from build123d import *

# Parameters (mm, degrees)
BOSS_EXTRUDE1_DEPTH = 12


with BuildPart() as part:
    # Sketch1 → Boss-Extrude1 (new body)
    with BuildSketch(Plane.XY):
        with BuildLine():
            Line((0.477214368, -2.672855337), (26.843355259, 7.215507779))
            ThreePointArc((26.843355259, 7.215507779), (36.953291517, 0.789364626), (27.989636176, -7.157899677))
            Line((27.989636176, -7.157899677), (15.076637928, -4.54511037))
            ThreePointArc((15.076637928, -4.54511037), (14.494851923, -4.485141012), (13.912410709, -4.538371753))
            Line((13.912410709, -4.538371753), (-14.128816251, -12.448152272))
            ThreePointArc((-14.128816251, -12.448152272), (-15.750958715, -12.635893161), (-17.350003272, -12.304759779))
            Line((-17.350003272, -12.304759779), (-32.894889614, -7.121812332))
            ThreePointArc((-32.894889614, -7.121812332), (-37.600806958, 2.472956777), (-27.935809428, 7.032899219))
            Line((-27.935809428, 7.032899219), (-1.504706088, -2.679457675))
            ThreePointArc((-1.504706088, -2.679457675), (-0.513152862, -2.854165557), (0.477214368, -2.672855337))
        make_face()
        with BuildLine():
            Line((-28.280719883, 6.094263625), (-1.849616543, -3.618093269))
            ThreePointArc((-1.849616543, -3.618093269), (-0.509821597, -3.854160008), (0.82837082, -3.609172135))
            Line((0.82837082, -3.609172135), (27.194511712, 6.279190981))
            ThreePointArc((27.194511712, 6.279190981), (35.956456468, 0.709866915), (28.187955173, -6.177762148))
            Line((28.187955173, -6.177762148), (15.274956925, -3.564972841))
            ThreePointArc((15.274956925, -3.564972841), (14.477361985, -3.485090396), (13.679767045, -3.564972841))
            Line((13.679767045, -3.564972841), (-14.400299195, -11.485709022))
            ThreePointArc((-14.400299195, -11.485709022), (-15.71642918, -11.636427946), (-17.012660358, -11.363116652))
            Line((-17.012660358, -11.363116652), (-32.578589422, -6.173153179))
            ThreePointArc((-32.578589422, -6.173153179), (-36.657051163, 2.142313468), (-28.280719883, 6.094263625))
        make_face(mode=Mode.SUBTRACT)
    extrude(amount=BOSS_EXTRUDE1_DEPTH)


solid = part.part
Source: CAD feature listing. Evaluate the final solid. Frame: model axes, mm. A direction names the side the tool comes from. Give positions to 0.01 mm unless a question says otherwise; leave off trailing zeros. Write each loop counter-clockwise with the first axis right and the second up, starting at its lowest first coordinate (ties: lowest second). Pieces come first, ordered by that corner, then holes. Notation, with made-up numbers: (71, -28) -> (103, -28) arc R22 ccw to (103, -2) -> close; hole circle Ø2 at (60.5, 3). An arc over 180 degrees is marked (long way). Return JSON: item names as keys, results as strings. Group by question number.
1. Material intervals for line 1 (Y direction, x = 6, z = 1); line 2 (Y direction, x = -19, z = 10.5), sorted ascending. Write a range as from..to.
2. Section C-C, the plane x = 1.5. Output: boundary loops of the cut face in (y, z).
3. Access query for faces 4 (the face through (-15.25, 1.306, 5.916)), 5 (the face through (0.088, -8.438, 5.916)), 6 (the face through (13.476, 2.202, 5.916)). Directions: +Z, -Z, +X, -X, +Y, -Y. A direction counts if a zero-diameter tool reaches every point of the face in a straight line with its end or side. Return the directions, or none.
4. Section B-B, the plane y = 3.25. Output: boundary loops of the cut face in (x, z), then the cut area to 3 significant figures.
5. Pin query (flat end, axial travel): pin 1 Ø8 at (x, y) = (-27, -4) entering from +Z; pin 2 Ø6 at (x, z) = (8.5, 10.5) entering from +Y; pin 3 Ø6 at (y, z) = (-6.5, 10.5) entering from +X; pin 4 Ø1.5 at (y, z) = (4.5, 7.5) entering from -X. Return the tip coordinate at first contact, or that it passes through.
6. Section D-D, the plane y = -8. Output: boundary loops of the cut face in (x, z).
7. Mould query, pull axis Y, two halves, no side actions, for faces 1 (the face through (-15.728, -12.637, 5.916)), 2 (the face through (14.489, -3.485, 5.916)), 3 (the face through (-14.905, 2.245, 5.916)). Classes: +Y half, -Y half, draft (parallel to the pull), parting line (faces both ways), or undercut.
8. Section A-A, the plane z = 5.75. Output: boundary loops of the cut face in (x, y), then the cut area to 3 significant figures.
Determined:
{
 "1": {"line 1": "y = -6.77..-5.73, -1.67..-0.6", "line 2": "y = -11.75..-10.7, 2.68..3.75"},
 "2": {"outline": "(-8.04, 0) -> (-7, 0) -> (-7, 12) -> (-8.04, 12) -> close; (-3.36, 0) -> (-2.29, 0) -> (-2.29, 12) -> (-3.36, 12) -> close"},
 "3": {"face 4": "+Z, -Z", "face 5": "+Z, -Z, -Y", "face 6": "+Z, -Z, +Y"},
 "4": {"outline": "(-37.28, 0) -> (-36.15, 0) -> (-36.15, 12) -> (-37.28, 12) -> close; (-20.54, 0) -> (-17.64, 0) -> (-17.64, 12) -> (-20.54, 12) -> close; (16.27, 0) -> (19.12, 0) -> (19.12, 12) -> (16.27, 12) -> close; (35.21, 0) -> (36.33, 0) -> (36.33, 12) -> (35.21, 12) -> close", "area": "95.9 mm2"},
 "5": {"pin 1": "stops at z = 12", "pin 2": "stops at y = 1.46", "pin 3": "stops at x = 36", "pin 4": "stops at x = -37.01"},
 "6": {"outline": "(-30.26, 0) -> (-27.1, 0) -> (-27.1, 12) -> (-30.26, 12) -> close; (-2.04, 0) -> (1.64, 0) -> (1.64, 12) -> (-2.04, 12) -> close"},
 "7": {"face 1": "-Y half", "face 2": "undercut", "face 3": "+Y half"},
 "8": {"outline": "(-32.89, -7.12) -> (-17.35, -12.3) arc R5.13 ccw to (-14.13, -12.45) -> (13.91, -4.54) arc R3.02 cw to (15.08, -4.55) -> (27.99, -7.16) arc R7.5 ccw (long way) to (26.84, 7.22) -> (0.48, -2.67) arc R2.85 cw to (-1.5, -2.68) -> (-27.94, 7.03) arc R7.5 ccw (long way) to start; hole (-32.58, -6.17) -> (-17.01, -11.36) arc R4.13 ccw to (-14.4, -11.49) -> (13.68, -3.56) arc R4.02 cw to (15.27, -3.56) -> (28.19, -6.18) arc R6.5 ccw (long way) to (27.19, 6.28) -> (0.83, -3.61) arc R3.85 cw to (-1.85, -3.62) -> (-28.28, 6.09) arc R6.5 ccw (long way) to start", "area": "170 mm2"}
}
